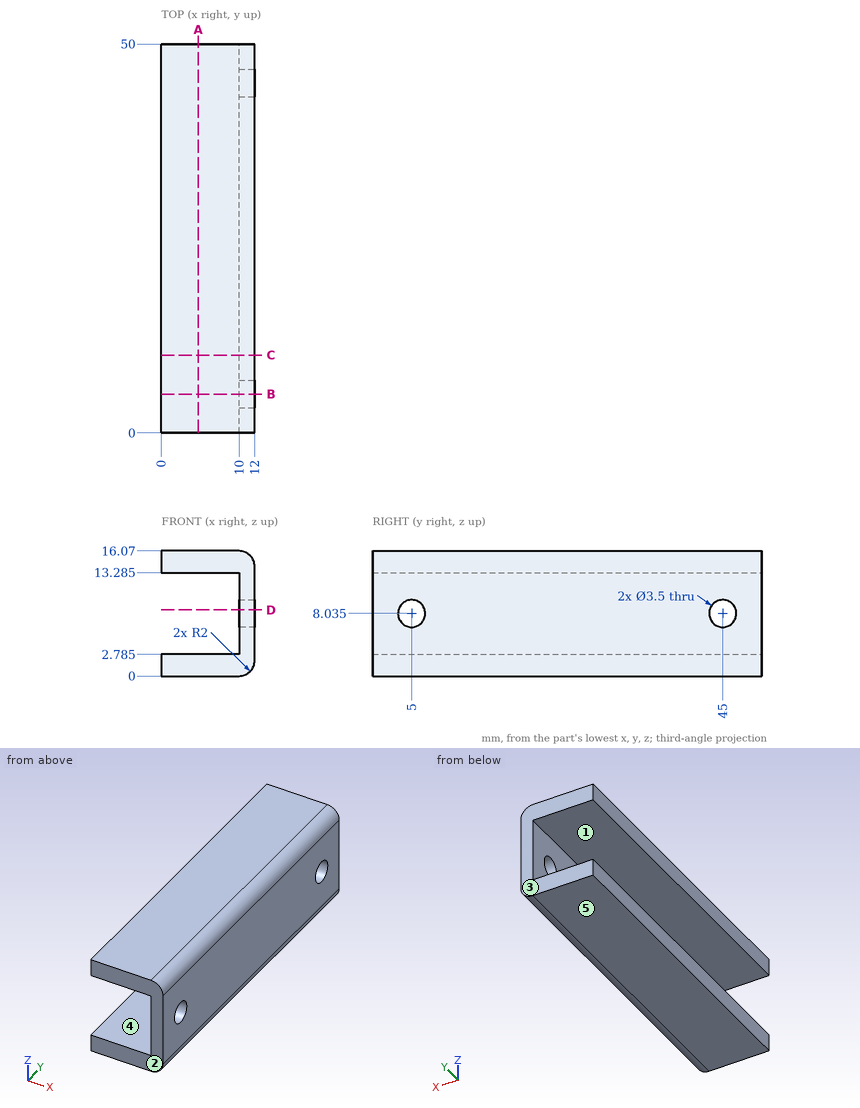
The figure shows three views and two pictorial views of one solid part (mm, origin at its lowest corner). Answer the questions. A direction names the side the tool comes from. Give positions to 0.01 mm unless a question says otherwise; leave off trailing zeros. Write each loop counter-clockwise with the first axis right and the second up, starting at its lowest first coordinate (ties: lowest second). Pieces come first, ordered by that corner, then holes. Notation, with made-up numbers: (-25, -28) -> (4, -28) arc R29 ccw to (4, -2) -> close; hole circle Ø6 at (-21.5, 58.5). An arc over 180 degrees is marked (long way). Answer as a JSON object with one key per item and string values.
1) Straight lines are drawn through the part: probe 1 along Z at (x, y) = (7.25, 17) (3 decimals); probe 2 along X at (y, z) = (20.5, 12.75); probe 3 along Y at (x, z) = (10.75, 7). For each, find the intervals that lie inside material, in ascending order. Write a range as from..to.
Findings below:
{"probe 1": "z = 0..2.785, 13.285..16.07", "probe 2": "x = 10..12", "probe 3": "y = 0..3.59, 6.41..43.59, 46.41..50"}
2) A tool of negligible diameter and unlimited length cuts with its end or side. For the marked faces 1 and 2, from which of +Z, -Z, +X, -X, +Y, -Y can it reach the whole face along a straight path? Write none if from no direction.
Findings below:
{"face 1": "-X, +Y, -Y", "face 2": "+Z, -Z, +X, -X, -Y"}
3) Section A-A on x = 4.75 is taken. Write down the section's boundary in (y, z) (3 decimals).
Findings below:
{"outline": "(0, 0) -> (50, 0) -> (50, 2.785) -> (0, 2.785) -> close; (0, 13.285) -> (50, 13.285) -> (50, 16.07) -> (0, 16.07) -> close"}
4) For a pull along Z with two mould halves and no side action, classify the marked faces 3, 4 and 5 as pulls with the +Z half, pulls with the -Z half, needs draft (parallel to the pull), parting line crosses it, or undercut.
Findings below:
{"face 3": "needs draft", "face 4": "undercut", "face 5": "pulls with the -Z half"}
5) Section B-B on y = 5 is taken. Write down the section's boundary in (x, z) (3 decimals), then the cut area to 3 significant figures.
Findings below:
{"outline": "(0, 0) -> (10, 0) arc R2 ccw to (12, 2) -> (12, 6.285) -> (10, 6.285) -> (10, 2.785) -> (0, 2.785) -> close; (0, 13.285) -> (10, 13.285) -> (10, 9.785) -> (12, 9.785) -> (12, 14.07) arc R2 ccw to (10, 16.07) -> (0, 16.07) -> close", "area": "79.1 mm^2"}
6) A flat-ended cylindrical pin translates along its axis: pin 1 Ø5 at (y, z) = (33, 7.5) entering from -X. Find the tip coordinate at first contact, or state that the pin passes through.
Findings below:
{"pin 1": "stops at x = 10"}
7) Section C-C on y = 10 is taken. Write down the section's boundary in (x, z) (3 decimals).
Findings below:
{"outline": "(0, 0) -> (10, 0) arc R2 ccw to (12, 2) -> (12, 14.07) arc R2 ccw to (10, 16.07) -> (0, 16.07) -> (0, 13.285) -> (10, 13.285) -> (10, 2.785) -> (0, 2.785) -> close"}
8) Section D-D on z = 8.5 is taken. Write down the section's boundary in (x, y), then the cut area to 3 significant figures.
Findings below:
{"outline": "(10, 0) -> (12, 0) -> (12, 3.31) -> (10, 3.31) -> close; (10, 6.69) -> (12, 6.69) -> (12, 43.31) -> (10, 43.31) -> close; (10, 46.69) -> (12, 46.69) -> (12, 50) -> (10, 50) -> close", "area": "86.5 mm^2"}
